from build123d import *

# Parameters (mm, degrees)
SKETCH_1_R          = 18.5
SKETCH_1_R_2        = 2.1
SKETCH_1_R_3        = 6.35
EXTRUDE_1_DEPTH     = 43
SKETCH_2_R          = 18.5
CUT_EXTRUDE_1_DEPTH = 40
SKETCH_3_R          = 1.5
CUT_EXTRUDE_2_DEPTH = 40
SKETCH_4_R          = 1.5
CUT_EXTRUDE_3_DEPTH = 100


with BuildPart() as part:
    # Эскиз1 → Бобышка-Вытянуть1 (new body)
    # profile 1 of 2: a face of its own
    with BuildSketch(Plane.XY):
        with BuildLine():
            Line((30, -18.5), (18.901833927, 7.935406367))
            ThreePointArc((18.901833927, 7.935406367), (0, 20.5), (-18.901833927, 7.935406367))
            Line((-18.901833927, 7.935406367), (-30, -18.5))
            Line((-30, -18.5), (-30, -20.5))
            Line((-30, -20.5), (0, -20.5))
            Line((0, -20.5), (30, -20.5))
            Line((30, -20.5), (30, -18.5))
        make_face()
        Circle(SKETCH_1_R, mode=Mode.SUBTRACT)
    # profile 2 of 2: a face of its own
    with BuildSketch(Plane.XY):
        Circle(SKETCH_1_R)
        with Locations((7.75, 13.423393759)):
            Circle(SKETCH_1_R_2, mode=Mode.SUBTRACT)
        with Locations((-7.75, 13.423393759)):
            Circle(SKETCH_1_R_2, mode=Mode.SUBTRACT)
        with Locations((-15.5, 0)):
            Circle(SKETCH_1_R_2, mode=Mode.SUBTRACT)
        with Locations((-7.75, -13.423393759)):
            Circle(SKETCH_1_R_2, mode=Mode.SUBTRACT)
        with Locations((7.75, -13.423393759)):
            Circle(SKETCH_1_R_2, mode=Mode.SUBTRACT)
        with Locations((15.5, 0)):
            Circle(SKETCH_1_R_2, mode=Mode.SUBTRACT)
        with Locations((0, 7)):
            Circle(SKETCH_1_R_3, mode=Mode.SUBTRACT)
    extrude(amount=EXTRUDE_1_DEPTH)

    # Эскиз2 → Вырез-Вытянуть1 (cut)
    with BuildSketch(Plane.XY.offset(43)):
        Circle(SKETCH_2_R)
    extrude(amount=-CUT_EXTRUDE_1_DEPTH, mode=Mode.SUBTRACT)

    # Эскиз3 → Вырез-Вытянуть2 (cut)
    with BuildSketch(Plane(origin=(0, -20.5, 0), x_dir=(-1, 0, 0), z_dir=(0, -1, 0))):
        with Locations(Location((25, -38, 0), (0, 0, 90))):
            Circle(SKETCH_3_R)
        with Locations(Location((25, -21.5, 0), (0, 0, 90))):
            Circle(SKETCH_3_R)
        with Locations(Location((25, -5, 0), (0, 0, 90))):
            Circle(SKETCH_3_R)
        with Locations(Location((-25, -38, 0), (0, 0, 90))):
            Circle(SKETCH_3_R)
        with Locations(Location((-25, -21.5, 0), (0, 0, 90))):
            Circle(SKETCH_3_R)
        with Locations(Location((-25, -5, 0), (0, 0, 90))):
            Circle(SKETCH_3_R)
    extrude(amount=-CUT_EXTRUDE_2_DEPTH, mode=Mode.SUBTRACT)

    # Эскиз4 → Вырез-Вытянуть3 (cut)
    with BuildSketch(Plane(origin=(0, -20.5, 0), x_dir=(-1, 0, 0), z_dir=(0, -1, 0))):
        with Locations(Location((0, -21.5, 0), (0, 0, 90))):
            Circle(SKETCH_4_R)
    extrude(amount=-CUT_EXTRUDE_3_DEPTH, mode=Mode.SUBTRACT)


solid = part.part
The listing builds one solid part. Answer for the finished solid, in the listing's coordinates (mm). A direction names the side the tool comes from. Coordinates: 2 decimals unless noted, no trailing zeros. Write each loop counter-clockwise with the first axis right and the second up, starting at its lowest first coordinate (ties: lowest second). Pieces come first, ordered by that corner, then holes. Notation, with made-up numbers: (5, 11) - (63, 11) arc R18 cw to (63, 18) - close; hole circle Ø7 at (-1.75, 43.5). An arc over 180 degrees is marked (long way). Return JSON: item names as keys, results as strings.
1. Each of these flat-tipped pins is pushed along its axis until it touches: pin 1 Ø3.5 at (x, y) = (-7.75, -13.42) entering from +Z; pin 2 Ø3 at (x, y) = (-9, 0) entering from +Z; pin 3 Ø1.5 at (y, z) = (0.5, 18.5) entering from -X; pin 4 Ø8 at (y, z) = (0, 20) entering from +X. Where does it stop, or does it pass through?
Final values:
{"pin 1": "through", "pin 2": "z = 3", "pin 3": "x = -22.34", "pin 4": "x = 23.91"}
2. Consider line 1 along Z through (x, y) = (25, -12); line 2 along Z through (x, y) = (24, -9); line 3 along Z through (x, y) = (1, -18). Determine where each line is inside the solid, lowest interval first.
Final values:
{"line 1": "0 to 3.5, 6.5 to 20, 23 to 36.5, 39.5 to 43", "line 2": "0 to 3.88, 6.12 to 20.38, 22.62 to 36.88, 39.12 to 43", "line 3": "0 to 3"}
3. Which of the six approach directions +Z, -Z, +X, -X, +Y, -Y give full straight-line access (tool end or side, diameter ignored) to faces 1 (the face through (-4.01, -18.06, 23.28)), 2 (the face through (23.67, -13.79, 4.31))?
Final values:
{"face 1": "+Z", "face 2": "+Y, -Y"}
4. For a pull along Z with two mould halves and no side action, classify faces 3 (the face through (0, 0, 3)), 4 (the face through (0, 19, 23)), 5 (the face through (-1.38, 0.8, 1.48)) as +Z half, -Z half, draft (parallel to the pull), parting line (faces both ways), or undercut.
Final values:
{"face 3": "+Z half", "face 4": "undercut", "face 5": "draft"}
5. The part is cut by section B-B on x = 0. Determine the outline of the cut face in (y, z), then the cut area to 3 significant figures.
Final values:
{"outline": "(-20.5, 0) - (0.65, 0) - (0.65, 3) - (-18.5, 3) - (-18.5, 20) - (-20.5, 20) - close; (-20.5, 23) - (-18.5, 23) - (-18.5, 43) - (-20.5, 43) - close; (13.35, 0) - (20.5, 0) - (20.5, 20) - (18.5, 20) - (18.5, 3) - (13.35, 3) - close; (18.5, 23) - (20.5, 23) - (20.5, 43) - (18.5, 43) - close", "area": "233 mm^2"}
6. The part is cut by section A-A on z = 5. Determine the outline of the cut face in (x, y), then the cut area to 3 significant figures.
Final values:
{"outline": "(-30, -20.5) - (-26.5, -20.5) - (-26.5, -10.16) - (-30, -18.5) - close; (-23.5, -20.5) - (23.5, -20.5) - (23.5, -3.02) - (18.9, 7.94) arc R20.5 ccw to (-18.9, 7.94) - (-23.5, -3.02) - close; (26.5, -20.5) - (30, -20.5) - (30, -18.5) - (26.5, -10.16) - close; hole circle Ø37 at (0, 0)", "area": "597 mm^2"}
7. The part is cut by section C-C on z = 21.5. Determine the outline of the cut face in (x, y).
Final values:
{"outline": "(-30, -20.5) - (-26.5, -20.5) - (-26.5, -10.16) - (-30, -18.5) - close; (-23.5, -20.5) - (-1.5, -20.5) - (-1.5, -18.44) arc R18.5 cw to (-1.5, 18.44) - (-1.5, 20.45) arc R20.5 ccw to (-18.9, 7.94) - (-23.5, -3.02) - close; (1.5, -20.5) - (23.5, -20.5) - (23.5, -3.02) - (18.9, 7.94) arc R20.5 ccw to (1.5, 20.45) - (1.5, 18.44) arc R18.5 cw to (1.5, -18.44) - close; (26.5, -20.5) - (30, -20.5) - (30, -18.5) - (26.5, -10.16) - close"}
8. The part is cut by section D-D on y = -17. Determine the outline of the cut face in (x, z).
Final values:
{"outline": "(-29.37, 0) - (29.37, 0) - (29.37, 43) - (7.3, 43) - (7.3, 3) - (-7.3, 3) - (-7.3, 43) - (-29.37, 43) - close; hole circle Ø3 at (-25, 5); hole circle Ø3 at (-25, 21.5); hole circle Ø3 at (-25, 38); hole circle Ø3 at (25, 5); hole circle Ø3 at (25, 21.5); hole circle Ø3 at (25, 38)"}
